Input: part model. Units: mm. Frame: model coordinates. A direction names the side the tool comes from. Coordinates: 2 decimals unless noted, no trailing zeros. Loops run counter-clockwise (first coordinate to the right, second up) from the corner with the lowest first, then second, coordinate; pieces in that order, holes last. Notation, with made-up numbers: M -6,88.5 L 14,88.5 A22 cw 14,115.5 Z; hole C -9,22 d10. An arc over 180 degrees is marked long. Use a Markdown table: item, result. Add a question column.
1. Section B-B on x = 39. State how many separate pieces and enclosed holes the cut face has, then the cut area to 3 significant figures.
2. Set-up query: faces 1 (the flat face through (-1, 1.5, 5)), 2 (the flat face through (0, 3, -3.797)), 3 (the cylindrical face through (-0.325, 0.76, -5.286)). Return all of +Z, -Z, +X, -X, +Y, -Y with unobstructed straight access to the full face (end or side cutting, diameter ignored); none if empty.
3. Section A-A on y = 26. Output: boundary loops of the cut face in (x, z), then the cut area to 3 significant figures.
4. Draft query along X for faces 4 (the cylindrical face through (37.81, 0.76, 7.66)), 5 (the flat face through (38, 24, -19)). Return one class per face: +X half, -X half, draft (parallel to the pull), parting line (faces both ways), or undercut.
5. Pin query (flat end, axial travel): pin 1 (11.5 mm diameter, centred on x = 19.5, y = 21, fed in from +Z); pin 2 (1 mm diameter, centred on x = 22, z = -12.5, fed in from -Y); pin 3 (6.5 mm diameter, centred on x = 37.5, z = 7, fed in from +Y). Return the tip coordinate at first contact, or that it passes through.
6. Section D-D on y = 16. Output: boundary loops of the cut face in (x, z).
7. Section C-C on z = 4.5. Output: boundary loops of the cut face in (x, y), then the cut area to 3 significant figures.
8. Line query: L1, parallel to X at y = 1.1, z = 6.75; L2, parallel to Z at x = 39, y = 1; L3, parallel to Z at x = 0.5, y = 2. Output: solid intervals per line, ascending. Write a range as [from, to].
```python
from build123d import *

# Parameters (mm, degrees)
SKETCH1_W           = 8.5
SKETCH1_H           = 22
BOSS_EXTRUDE1_DEPTH = 5
CUT_EXTRUDE1_DEPTH  = 3.5
SKETCH3_R           = 1.5
CUT_EXTRUDE2_DEPTH  = 1.5
SKETCH4_W           = 8.5
SKETCH4_H           = 6
BOSS_EXTRUDE2_DEPTH = 23
SKETCH7_W           = 8.5
SKETCH7_H           = 22
BOSS_EXTRUDE4_DEPTH = 5
CUT_EXTRUDE3_DEPTH  = 3.5
SKETCH9_R           = 1.5
CUT_EXTRUDE4_DEPTH  = 3.5
SKETCH10_W          = 8.5
SKETCH10_H          = 6
BOSS_EXTRUDE5_DEPTH = 23
SKETCH6_W           = 6
SKETCH6_H           = 8
BOSS_EXTRUDE6_DEPTH = 30.5
SKETCH11_W          = 47.5
SKETCH11_H          = 8
BOSS_EXTRUDE7_DEPTH = 13.5
SKETCH12_W          = 47.5
SKETCH12_H          = 8
BOSS_EXTRUDE8_DEPTH = 5.5
SKETCH13_W          = 5
SKETCH13_H          = 6
CUT_EXTRUDE5_DEPTH  = 15
SKETCH14_W          = 5
SKETCH14_H          = 6
CUT_EXTRUDE6_DEPTH  = 4
SKETCH15_W          = 5
SKETCH15_H          = 6
CUT_EXTRUDE7_DEPTH  = 15
SKETCH16_W          = 5
SKETCH16_H          = 6
CUT_EXTRUDE8_DEPTH  = 4


with BuildPart() as part:
    # Sketch1 → Boss-Extrude1 (new body)
    with BuildSketch(Plane(origin=(0, 0, 0), x_dir=(1, 0, 0), z_dir=(0, 1, 0))):
        Rectangle(SKETCH1_W, SKETCH1_H)
    extrude(amount=BOSS_EXTRUDE1_DEPTH)

    # Sketch2 → Cut-Extrude1 (cut)
    with BuildSketch(Plane(origin=(0, 5, 0), x_dir=(1, 0, 0), z_dir=(0, 1, 0))):
        Polygon((-1.705, 9.703146627), (-3.41, 6.75), (-1.705, 3.796853373), (1.705, 3.796853373), (3.41, 6.75), (1.705, 9.703146627), align=None)
        Polygon((1.705, -9.703146627), (-1.705, -9.703146627), (-3.41, -6.75), (-1.705, -3.796853373), (1.705, -3.796853373), (3.41, -6.75), align=None)
    extrude(amount=-CUT_EXTRUDE1_DEPTH, mode=Mode.SUBTRACT)

    # Sketch3 → Cut-Extrude2 (cut)
    with BuildSketch(Plane(origin=(0, 1.5, 0), x_dir=(1, 0, 0), z_dir=(0, 1, 0))):
        with Locations((0, 6.75)):
            Circle(SKETCH3_R)
        with Locations((0, -6.75)):
            Circle(SKETCH3_R)
        with Locations((39, 6.75)):
            Circle(SKETCH3_R)
        with Locations((39, -6.75)):
            Circle(SKETCH3_R)
    extrude(amount=-CUT_EXTRUDE2_DEPTH, mode=Mode.SUBTRACT)

    # Sketch4 → Boss-Extrude2 (add)
    with BuildSketch(Plane(origin=(0, 5, 0), x_dir=(1, 0, 0), z_dir=(0, 1, 0))):
        Rectangle(SKETCH4_W, SKETCH4_H)
    extrude(amount=BOSS_EXTRUDE2_DEPTH)



with BuildPart() as body_2:
    # Sketch7 → Boss-Extrude4 (new body)
    with BuildSketch(Plane(origin=(0, 0, 0), x_dir=(1, 0, 0), z_dir=(0, 1, 0))):
        with Locations((39, 0)):
            Rectangle(SKETCH7_W, SKETCH7_H)
    extrude(amount=BOSS_EXTRUDE4_DEPTH)

    # Sketch8 → Cut-Extrude3 (cut)
    with BuildSketch(Plane(origin=(0, 5, 0), x_dir=(1, 0, 0), z_dir=(0, 1, 0))):
        Polygon((40.705, 9.703146627), (37.295, 9.703146627), (35.59, 6.75), (37.295, 3.796853373), (40.705, 3.796853373), (42.41, 6.75), align=None)
        Polygon((40.705, -3.796853373), (37.295, -3.796853373), (35.59, -6.75), (37.295, -9.703146627), (40.705, -9.703146627), (42.41, -6.75), align=None)
    extrude(amount=-CUT_EXTRUDE3_DEPTH, mode=Mode.SUBTRACT)

    # Sketch9 → Cut-Extrude4 (cut)
    with BuildSketch(Plane(origin=(0, 1.5, 0), x_dir=(1, 0, 0), z_dir=(0, 1, 0))):
        with Locations((39, 6.75)):
            Circle(SKETCH9_R)
        with Locations((39, -6.75)):
            Circle(SKETCH9_R)
    extrude(amount=-CUT_EXTRUDE4_DEPTH, mode=Mode.SUBTRACT)

    # Sketch10 → Boss-Extrude5 (add)
    with BuildSketch(Plane(origin=(0, 5, 0), x_dir=(1, 0, 0), z_dir=(0, 1, 0))):
        with Locations((39, 0)):
            Rectangle(SKETCH10_W, SKETCH10_H)
    extrude(amount=BOSS_EXTRUDE5_DEPTH)


with BuildPart() as part_1:
    add(part.part)

    add(body_2.part)  # Boss-Extrude6 merges body 2
    # Sketch6 → Boss-Extrude6 (add)
    with BuildSketch(Plane(origin=(4.25, 0, 0), x_dir=(0, 0, -1), z_dir=(1, 0, 0))):
        with Locations((0, 24)):
            Rectangle(SKETCH6_W, SKETCH6_H)
    extrude(amount=BOSS_EXTRUDE6_DEPTH)

    # Sketch11 → Boss-Extrude7 (add)
    with BuildSketch(Plane(origin=(0, 0, -3), x_dir=(-1, 0, 0), z_dir=(0, 0, -1))):
        with Locations((-19.5, 24)):
            Rectangle(SKETCH11_W, SKETCH11_H)
    extrude(amount=BOSS_EXTRUDE7_DEPTH)

    # Sketch12 → Boss-Extrude8 (add)
    with BuildSketch(Plane(origin=(0, 0, -16.5), x_dir=(-1, 0, 0), z_dir=(0, 0, -1))):
        with Locations((-19.5, 24)):
            Rectangle(SKETCH12_W, SKETCH12_H)
    extrude(amount=BOSS_EXTRUDE8_DEPTH)

    # Sketch13 → Cut-Extrude5 (cut)
    with BuildSketch(Plane.ZY.offset(4.25)):
        with Locations((-16.5, 24)):
            Rectangle(SKETCH13_W, SKETCH13_H)
    extrude(amount=-CUT_EXTRUDE5_DEPTH, mode=Mode.SUBTRACT)

    # Sketch14 → Cut-Extrude6 (cut)
    with BuildSketch(Plane(origin=(0, 0, -22), x_dir=(-1, 0, 0), z_dir=(0, 0, -1))):
        with Locations((-8.25, 24)):
            Rectangle(SKETCH14_W, SKETCH14_H)
    extrude(amount=-CUT_EXTRUDE6_DEPTH, mode=Mode.SUBTRACT)

    # Sketch15 → Cut-Extrude7 (cut)
    with BuildSketch(Plane(origin=(43.25, 0, 0), x_dir=(0, 0, -1), z_dir=(1, 0, 0))):
        with Locations((16.5, 24)):
            Rectangle(SKETCH15_W, SKETCH15_H)
    extrude(amount=-CUT_EXTRUDE7_DEPTH, mode=Mode.SUBTRACT)

    # Sketch16 → Cut-Extrude8 (cut)
    with BuildSketch(Plane(origin=(0, 0, -22), x_dir=(-1, 0, 0), z_dir=(0, 0, -1))):
        with Locations((-30.75, 24)):
            Rectangle(SKETCH16_W, SKETCH16_H)
    extrude(amount=-CUT_EXTRUDE8_DEPTH, mode=Mode.SUBTRACT)


solid = part_1.part
```
Answers below:
| question | item | result |
|---|---|---|
| 1 | separate pieces | 3 |
| 1 | enclosed holes | 1 |
| 1 | area | 320 mm² |
| 2 | face 1 | +Y |
| 2 | face 2 | none |
| 2 | face 3 | -Y |
| 3 | outline | M -4.25,-22 L 5.75,-22 L 5.75,-19 L -4.25,-19 Z; M -4.25,-14 L 10.75,-14 L 10.75,-22 L 28.25,-22 L 28.25,-14 L 43.25,-14 L 43.25,3 L -4.25,3 Z; M 33.25,-22 L 43.25,-22 L 43.25,-19 L 33.25,-19 Z |
| 3 | area | 1,010 mm² |
| 4 | face 4 | undercut |
| 4 | face 5 | draft |
| 5 | pin 1 | stops at z = 3 |
| 5 | pin 2 | stops at y = 20 |
| 5 | pin 3 | stops at y = 5 |
| 6 | outline | M -4.25,-3 L 4.25,-3 L 4.25,3 L -4.25,3 Z; M 34.75,-3 L 43.25,-3 L 43.25,3 L 34.75,3 Z |
| 7 | outline | M -4.25,0 L 4.25,0 L 4.25,5 L 2.11,5 L 2.11,1.5 L -2.11,1.5 L -2.11,5 L -4.25,5 Z; M 34.75,0 L 43.25,0 L 43.25,5 L 41.11,5 L 41.11,1.5 L 36.89,1.5 L 36.89,5 L 34.75,5 Z |
| 7 | area | 55.4 mm² |
| 8 | L1 | x = [-4.25, -1.5], [1.5, 4.25], [34.75, 37.5], [40.5, 43.25] |
| 8 | L2 | z = [-11, -8.25], [-5.25, 5.25], [8.25, 11] |
| 8 | L3 | z = [-11, -9.7], [-3.8, 3.8], [9.7, 11] |
